```python
from build123d import *

# Parameters (mm, degrees)
SKETCH1_R           = 8.255
SKETCH1_R_2         = 6.35
BOSS_EXTRUDE1_DEPTH = 12.7
SKETCH2_R           = 8.255
BOSS_EXTRUDE2_DEPTH = 2.54
CHAMFER1_SIZE       = 0.508


with BuildPart() as part:
    # Sketch1 → Boss-Extrude1 (new body)
    with BuildSketch(Plane(origin=(0, 0, 0), x_dir=(1, 0, 0), z_dir=(0, 1, 0))):
        with Locations(Location((0, 0, 0), (0, 0, 270))):  # turned: the seam where the file's is
            Circle(SKETCH1_R)
        with Locations(Location((0, 0, 0), (0, 0, 270))):  # turned: the seam where the file's is
            Circle(SKETCH1_R_2, mode=Mode.SUBTRACT)
    extrude(amount=BOSS_EXTRUDE1_DEPTH)

    # Sketch2 → Boss-Extrude2 (add)
    with BuildSketch(Plane(origin=(0, 12.7, 0), x_dir=(1, 0, 0), z_dir=(0, 1, 0))):
        with Locations(Location((0, 0, 0), (0, 0, 270))):  # turned: the seam where the file's is
            Circle(SKETCH2_R)
    extrude(amount=BOSS_EXTRUDE2_DEPTH)

    # Chamfer1
    chamfer1_edges = [part.edges().sort_by_distance(p)[0] for p in [
        (0, 0, -6.35),
    ]]
    chamfer(chamfer1_edges, length=CHAMFER1_SIZE)


solid = part.part
```
Source: CAD feature listing. Evaluate the final solid. Frame: model axes, mm. Coordinates: 2 decimals unless noted, no trailing zeros. Order: outer loops, then holes, each group sorted by start corner. A loop starts at its lowest first (then second) coordinate and runs counter-clockwise, first axis right, second up. Notation, with made-up numbers: (72.25, -1) - (78.25, -1) arc R22 cw to (78.25, 6) - close; hole circle Ø10 at (44, 19.25). An arc over 180 degrees is marked (long way). One line per item, written item: value.
1) Cut plane A-A on x = 0. Output: boundary loops of the cut face in (y, z) (3 decimals), plus the area to 3 significant figures.
Computed values:
outline: (0, -8.255) - (15.24, -8.255) - (15.24, 8.255) - (0, 8.255) - (0, 6.858) - (0.508, 6.35) - (12.7, 6.35) - (12.7, -6.35) - (0.508, -6.35) - (0, -6.858) - close
area: 90.1 mm^2
2) Cut plane C-C on y = 9. Output: boundary loops of the cut face in (x, z) (3 decimals), plus the area to 3 significant figures.
Computed values:
outline: circle Ø16.51 at (0, 0); hole circle Ø12.7 at (0, 0)
area: 87.4 mm^2
3) Contact query for flat-ended pins moving along their axis: pin 1 (2 mm diameter, centred on y = 4.5, z = 5, fed in from +X); pin 2 (1 mm diameter, centred on x = 6.5, y = 13.5, fed in from -Z); pin 3 (2 mm diameter, centred on x = -3, y = 4.5, fed in from +Z). Output: stop coordinate, or through.
Computed values:
pin 1: stops at x = 7.22
pin 2: stops at z = -5.67
pin 3: stops at z = 8.01
4) Mould query, pull axis Z, two halves, no side actions, for faces 1 (the face through (-3.86, 6.52, -5.04)), 2 (the face through (0, 12.7, 0)), 3 (the face through (7, 0, 1)), 4 (the face through (-5.023, 7.513, -6.551)). Classes: released by +Z, released by -Z, zero draft, split by the parting line, or undercut.
Computed values:
face 1: undercut
face 2: undercut
face 3: zero draft
face 4: split by the parting line
5) Cut plane B-B on z = 0. Output: boundary loops of the cut face in (x, y) (3 decimals), plus the area to 3 significant figures.
Computed values:
outline: (-8.255, 0) - (-6.858, 0) - (-6.35, 0.508) - (-6.35, 12.7) - (6.35, 12.7) - (6.35, 0.508) - (6.858, 0) - (8.255, 0) - (8.255, 15.24) - (-8.255, 15.24) - close
area: 90.1 mm^2
6) Ray query, line 1 (X direction, y = 7.5, z = -0.25); line 2 (Y direction, x = 3.5, z = -0.5); line 3 (Z direction, x = 3.25, y = 9). Return the intervals inside material, ascending. Write a range as [from, to].
Computed values:
line 1: x = [-8.25, -6.35], [6.35, 8.25]
line 2: y = [12.7, 15.24]
line 3: z = [-7.59, -5.46], [5.46, 7.59]
